CAD build for the part. Positions are in the model's coordinates, mm. Give positions to 0.01 mm unless a question says otherwise; leave off trailing zeros. Order: outer loops, then holes, each group sorted by start corner. A loop starts at its lowest first (then second) coordinate and runs counter-clockwise, first axis right, second up. Notation, with made-up numbers: (-18, -40) -> (19, -40) arc R20 ccw to (19, -15) -> close; hole circle Ø8 at (-32, 44). An arc over 180 degrees is marked (long way). Use one line per item in the form item = value. Start each with the question number.
1) Cut at B-B, the plane y = 0. Give the cut face in (x, z) (1 decimal).
2) Mould opens along Y. For faces 1 (the face through (35, 2, 0)), 2 (the face through (-66.85, 80.42, -1.61)), 3 (the face through (-66.182, -79.625, -1.61)) say: pulls with the +Y half, pulls with the -Y half, needs draft (parallel to the pull), parting line crosses it, or undercut.
3) Probe line 1 (Y direction, x = -63.5, z = -2.2); line 2 (X direction, y = -84, z = -2.1); line 3 (X direction, y = 0, z = -2.2). List the from-to ranges inside material, lowest first.
4) Cut at C-C, the plane z = -2.3. State how many separate pieces and enclosed holes the cut face has, and give its area (3 significant figures).
5) Cut at A-A, the plane x = 184.15. Give the cut face in (y, z) (1 decimal).
Autodesk Inventor part; units mm, degrees
ref_plane "YZ Plane" through (0, 0, 0) normal (1, 0, 0) x (0, 1, 0)
ref_plane "XZ Plane" through (0, 0, 0) normal (0, 1, 0) x (-1, 0, 0)
ref_plane "XY Plane" through (0, 0, 0) normal (0, 0, 1) x (1, 0, 0)
sketch "Sketch1" plane through (0, 0, 0) normal (0, 0, 1) x (1, 0, 0)
  line L0 (-139.7, 114.3) -> (317.5, 114.3)
  line L1 (317.5, 114.3) -> (317.5, -114.3)
  line L2 (317.5, -114.3) -> (-139.7, -114.3)
  line L3 (-139.7, -114.3) -> (-139.7, 114.3)
  point P0 (0, 0)
  dimension "d0" = 457.2
  dimension "d1" = 228.6
  dimension "d2" = 114.3
  dimension "d3" = 139.7
extrude "Extrusion1" add sketch "Sketch1" against normal blind 3.175
hole "Hole1" at (184.15, 0, 0) direction (0, 0, -1) diameter 212.725 depth 25.4 tip angle 118
hole "Hole2" at (-63.5, 82.55, 0) direction (0, 0, -1) diameter 7.9375 depth 25.4 tip angle 118
hole "Hole3" at (-63.5, -82.55, 0) direction (0, 0, -1) diameter 7.9375 depth 25.4 tip angle 118
hole "Hole4" at (73.025, 82.55, 0) direction (0, 0, -1) diameter 7.9375 depth 25.4 tip angle 118
hole "Hole5" at (73.025, -82.55, 0) direction (0, 0, -1) diameter 6.35 depth 25.4 tip angle 118
hole "Hole6" at (279.4, 82.55, 0) direction (0, 0, -1) diameter 7.9375 depth 25.4 tip angle 118
hole "Hole7" at (279.4, -82.55, 0) direction (0, 0, -1) diameter 7.9375 depth 25.4 tip angle 118
properties part number "Fore_Base"
Result:
q1.outline = (-139.7, -3.2) -> (77.8, -3.2) -> (77.8, 0) -> (-139.7, 0) -> close; (290.5, -3.2) -> (317.5, -3.2) -> (317.5, 0) -> (290.5, 0) -> close
q2.face_1 = needs draft
q2.face_2 = undercut
q2.face_3 = undercut
q3.line_1 = -114.3 to -86.52, -78.58 to 78.58, 86.52 to 114.3
q3.line_2 = -139.7 to -67.19, -59.81 to 70.2, 75.85 to 118.9, 249.4 to 275.71, 283.09 to 317.5
q3.line_3 = -139.7 to 77.79, 290.51 to 317.5
q4.separate_pieces = 1
q4.enclosed_holes = 7
q4.area = 68,700 mm²
q5.outline = (-114.3, -3.2) -> (-106.4, -3.2) -> (-106.4, 0) -> (-114.3, 0) -> close; (106.4, -3.2) -> (114.3, -3.2) -> (114.3, 0) -> (106.4, 0) -> close
